Read the model definition and answer for the solid it produces. Units are mm, in the model's axes. A direction names the side the tool comes from. Give positions to 0.01 mm unless a question says otherwise; leave off trailing zeros. Write each loop counter-clockwise with the first axis right and the second up, starting at its lowest first coordinate (ties: lowest second). Pieces come first, ordered by that corner, then holes. Notation, with made-up numbers: M 57.25,50.5 L 74.25,50.5 A32 cw 74.25,82.5 Z; hole C 30,-19.75 d6. An arc over 180 degrees is marked long. Put each result on its own line as item: value.
from build123d import *

# Parameters (mm, degrees)
F0_R     = 3.982588
F1_DEPTH = 25.4


with BuildPart() as f1:
    # F0 (on Top) → F1 (new body)
    with BuildSketch(Plane.XY):
        with BuildLine():
            ThreePointArc((-10.250391, 8.447082), (-6.45395, 16.609431), (-10.250391, 24.77178))
            Line((-10.250391, 24.77178), (-10.250391, 38.438968))
            Line((-10.250391, 38.438968), (-3.900391, 38.438968))
            Line((-3.900391, 38.438968), (-3.900391, 8.067437))
            ThreePointArc((-3.900391, 8.067437), (-1.247671, 8.365105), (0, 10.724947))
            Line((0, 10.724947), (0, 39.125941))
            ThreePointArc((0, 39.125941), (-0.743949, 40.921993), (-2.54, 41.665941))
            Line((-2.54, 41.665941), (-20.310961, 41.665941))
            ThreePointArc((-20.310961, 41.665941), (-27.793714, 32.174841), (-20.310961, 22.68374))
            ThreePointArc((-20.310961, 22.68374), (-12.479962, 16.741734), (-17.126696, 8.07918))
            ThreePointArc((-17.126696, 8.07918), (-13.658499, 7.701584), (-10.250391, 8.447082))
        make_face()
        with Locations((-18.033097, 32.174841)):
            Circle(F0_R, mode=Mode.SUBTRACT)
    extrude(amount=F1_DEPTH)


solid = f1.part
(1) Section D-D on x = -25.5 is taken. Determine the outline of the cut face in (y, z), and give its area (3 significant figures).
Result:
outline: M 25.89,0 L 38.46,0 L 38.46,25.4 L 25.89,25.4 Z
area: 319 mm²
(2) Section C-C on z = 6 is taken. Determine the outline of the cut face in (x, y), and give its area (3 significant figures).
Result:
outline: M -20.31,22.68 A7.57 cw -17.13,8.08 A10.82 ccw -10.25,8.45 A10.67 ccw -10.25,24.77 L -10.25,38.44 L -3.9,38.44 L -3.9,8.07 A2.86 ccw 0,10.72 L 0,39.13 A2.54 ccw -2.54,41.67 L -20.31,41.67 A9.76 ccw Z; hole C -18.03,32.17 d7.97
area: 492 mm²
(3) Section B-B on x = -13.5 is taken. Determine the outline of the cut face in (y, z).
Result:
outline: M 7.71,0 L 11.05,0 L 11.05,25.4 L 7.71,25.4 Z; M 19.21,0 L 41.67,0 L 41.67,25.4 L 19.21,25.4 Z
(4) For a pull along Y with two mould halves and no side action, classify faces 4 (the face through (0, 25, 13)), 5 (the face through (-1.28, 8.343, 12.522)), 6 (the face through (-22.01, 32.35, 12.52)), 7 (the face through (-7, 38.439, 13)) as +Y half, -Y half, draft (parallel to the pull), parting line (faces both ways), or undercut.
Result:
face 4: draft
face 5: -Y half
face 6: undercut
face 7: undercut
(5) Straight lines are drawn through the part: line 1 along X through (y, z) = (29, 3.75); line 2 along X through (y, z) = (30, 16.5); line 3 along X through (y, z) = (27, 8.5). For each, find the intervals that lie inside material, in ascending order. Write a range as from..to.
Result:
line 1: x = -27.26..-20.44, -15.63..-10.25, -3.9..0
line 2: x = -27.55..-21.37, -14.7..-10.25, -3.9..0
line 3: x = -26.31..-10.25, -3.9..0
(6) Which of the six approach directions +Z, -Z, +X, -X, +Y, -Y give full straight-line access (tool end or side, diameter ignored) to faces 1 (the face through (-11, 41.666, 13)), 2 (the face through (-3.9, 23, 13)), 3 (the face through (-6.455, 16.479, 12.522))?
Result:
face 1: +Z, -Z, +X, -X, +Y
face 2: +Z, -Z, -Y
face 3: +Z, -Z
(7) Given pin 1 Ø7 at (x, z) = (-6.5, 6.5) entering from -Y; pin 2 Ø12.5 at (y, z) = (25.5, 8) entering from -X; pin 3 Ø1.5 at (y, z) = (16.5, 6) entering from -X, each flat-ended and moving along its own axis, determine where each tip first touches the part or whether it passes through.
Result:
pin 1: stops at y = 7.87
pin 2: stops at x = -27.78
pin 3: stops at x = -12.61
(8) Section A-A on y = 26 is taken. Determine the outline of the cut face in (x, z), and give its area (3 significant figures).
Result:
outline: M -25.59,0 L -10.25,0 L -10.25,25.4 L -25.59,25.4 Z; M -3.9,0 L 0,0 L 0,25.4 L -3.9,25.4 Z
area: 489 mm²
